Input: dimensioned drawing with shaded views. Units: mm. Origin: part minimum x, y, z. A direction names the side the tool comes from. Round coordinates to 2 decimals unless told otherwise and drop trailing zeros. Order: outer loops, then holes, each group sorted by start corner. A loop starts at its lowest first (then second) coordinate and runs counter-clockwise, first axis right, second up.
Item 1: Cut plane A-A on z = 4.35. Output: boundary loops of the cut face in (x, y).
Item 2: Reachability of the marked faces 4 and 5 from +Z, -Z, +X, -X, +Y, -Y: full face, straight path, thin tool, end or side. Return the list, or none.
Item 3: Cut plane B-B on y = 8.25. Output: boundary loops of the cut face in (x, z), then the cut area to 3 significant figures.
Item 4: Mould query, pull axis Y, two halves, no side actions, for the marked faces 1, 2 and 3. Classes: released by +Y, released by -Y, zero draft, split by the parting line, or undercut.
Item 5: First-contact query: pin 1 (3 mm diameter, centred on x = 5.5, z = 2.5, fed in from +Y); pin 2 (2 mm diameter, centred on y = 16, z = 4.5, fed in from -X); pin 3 (1.5 mm diameter, centred on y = 5, z = 3, fed in from +X); pin 4 (9 mm diameter, centred on x = 10, y = 12, fed in from +Z). Flat tips, straight axial feed; report the tip coordinate or a pass-through.
Item 6: Line query: L1, parallel to Y at x = 15, z = 3.45; L2, parallel to Y at x = 15, z = 1.85; L3, parallel to X at y = 23.5, z = 4.4. Output: solid intervals per line, ascending.
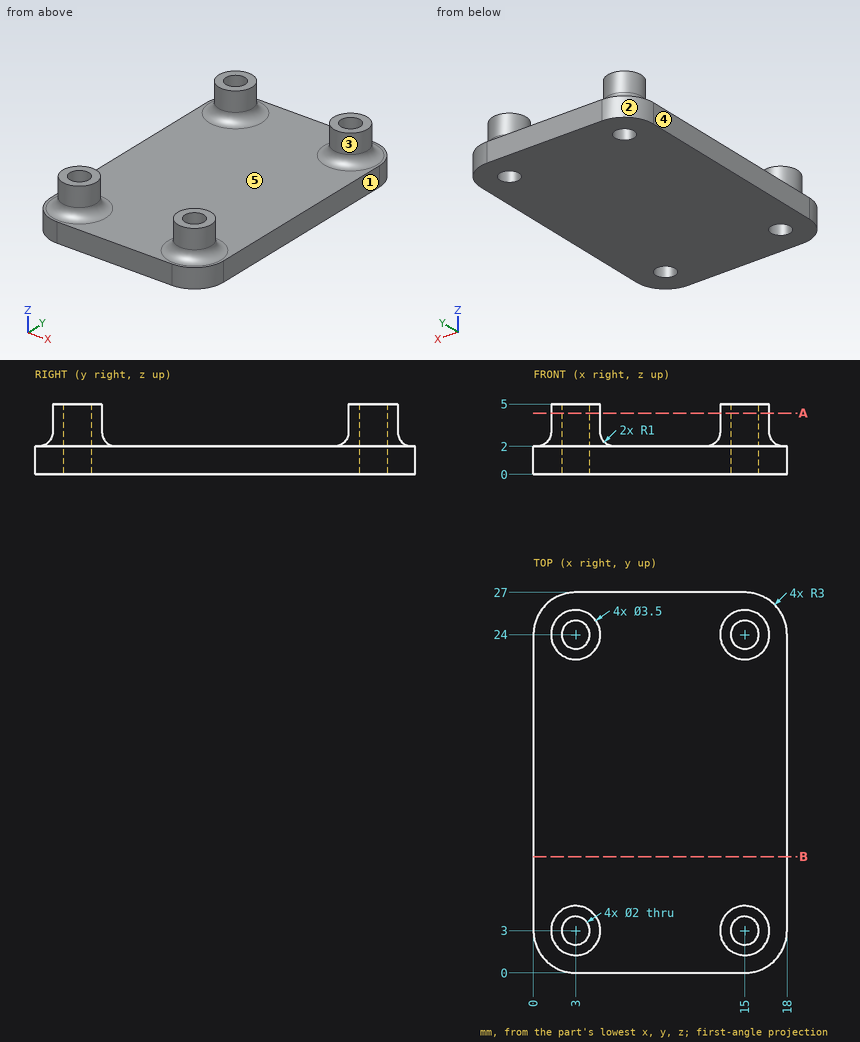
From the geometry:
1. outline: circle Ø3.5 at (3, 3); circle Ø3.5 at (3, 24); circle Ø3.5 at (15, 3); circle Ø3.5 at (15, 24); hole circle Ø2 at (3, 3); hole circle Ø2 at (3, 24); hole circle Ø2 at (15, 3); hole circle Ø2 at (15, 24)
2. face 4: +Z, -Z, -X, +Y, -Y
2. face 5: +Z
3. outline: (0, 0) - (18, 0) - (18, 2) - (0, 2) - close
3. area: 36.0 mm2
4. face 1: zero draft
4. face 2: released by +Y
4. face 3: undercut
5. pin 1: stops at y = 27
5. pin 2: passes through
5. pin 3: stops at x = 16.23
5. pin 4: stops at z = 2
6. L1: y = 1.25 to 2, 4 to 4.75, 22.25 to 23, 25 to 25.75
6. L2: y = 0 to 2, 4 to 23, 25 to 27
6. L3: x = 1.32 to 2.13, 3.87 to 4.68, 13.32 to 14.13, 15.87 to 16.68
